Can you work these out from the drawing? Everything is in mm from the part's minimum corner. Coordinates: 2 decimals unless noted, no trailing zeros. Order: outer loops, then holes, each group sorted by start corner. A loop starts at its lowest first (then second) coordinate and runs counter-clockwise, first axis right, second up. Notation, with made-up numbers: (44, -39) - (96, -39) arc R13 ccw to (96, -25) - close; hole circle Ø10 at (-36.5, -3). An arc over 180 degrees is marked (long way). Use a Markdown table: item, result. Add a question column.
(1) I want a section at C-C (y = 0.85). State how many separate pieces and enclosed holes the cut face has, and give its area (3 significant figures).
(2) I want a section at B-B (z = 113.5). List the corners of the cut face in (x, y) for me, and give its area (3 significant figures).
(3) I want a section at A-A (x = 207.5). List the corners of the cut face in (y, z) for me.
(4) If I drill on L1, parallel to Z at x = 7.5, y = 1.65; L2, parallel to X at y = 2.25, z = 70; L3, parallel to X at y = 1.55, z = 47.5, over which ranges is the centre line in solid material (lowest first)? Write a range as [from, to].
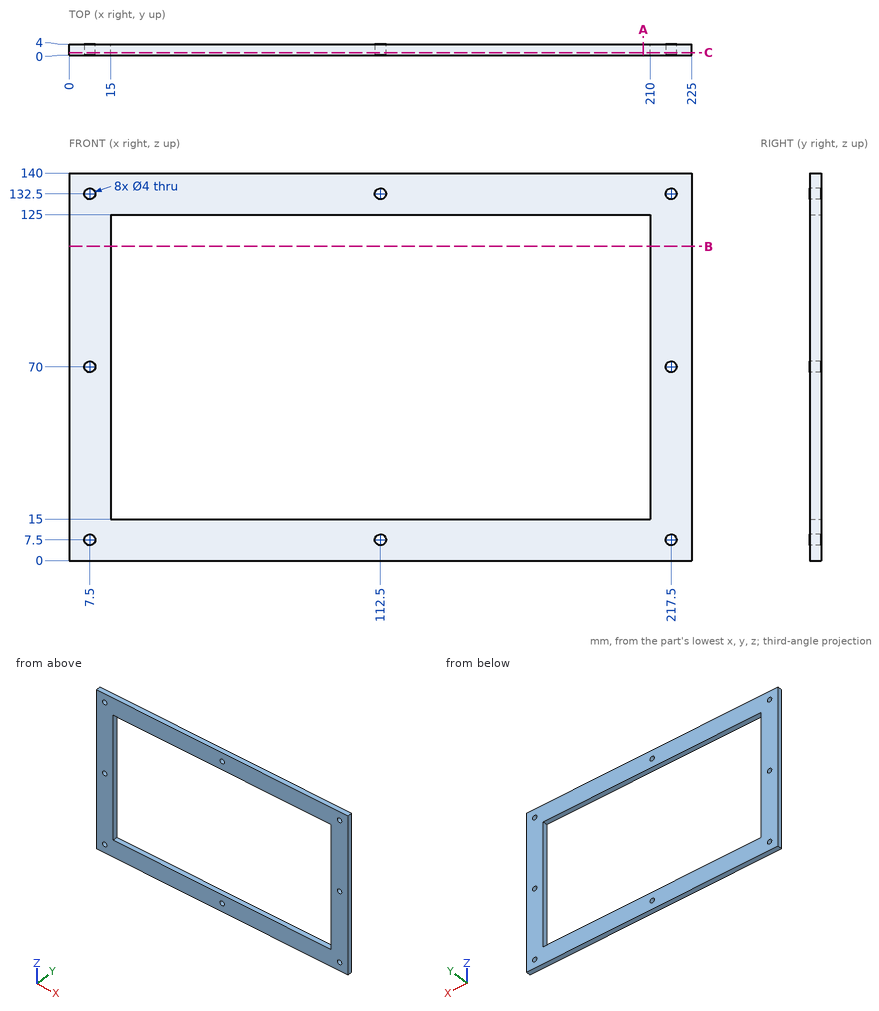
Answers follow:
| question | item | result |
|---|---|---|
| 1 | separate pieces | 1 |
| 1 | enclosed holes | 9 |
| 1 | area | 9,950 mm² |
| 2 | outline | (0, 0) - (15, 0) - (15, 4) - (0, 4) - close; (210, 0) - (225, 0) - (225, 4) - (210, 4) - close |
| 2 | area | 120 mm² |
| 3 | outline | (0, 0) - (4, 0) - (4, 15) - (0, 15) - close; (0, 125) - (4, 125) - (4, 140) - (0, 140) - close |
| 4 | L1 | z = [0, 5.5], [9.5, 68], [72, 130.5], [134.5, 140] |
| 4 | L2 | x = [0, 5.5], [9.5, 15], [210, 215.5], [219.5, 225] |
| 4 | L3 | x = [0, 15], [210, 225] |
